from build123d import *

# Parameters (mm, degrees)
SKETCH1_R           = 1.5
SKETCH1_W           = 13
SKETCH1_H           = 19.3
BOSS_EXTRUDE1_DEPTH = 1
FILLET1_R           = 3


with BuildPart() as part:
    # Sketch1 → Boss-Extrude1 (new, symmetric)
    with BuildSketch(Plane(origin=(0, 0, 0), x_dir=(1, 0, 0), z_dir=(0, 1, 0))):
        with BuildLine():
            Line((-105.5, 65), (-105.5, 69))
            ThreePointArc((-105.5, 69), (-109, 72.5), (-112.5, 69))
            Line((-112.5, 69), (-112.5, 65))
            Line((-112.5, 65), (-112.5, -65))
            Line((-112.5, -65), (-112.5, -69))
            ThreePointArc((-112.5, -69), (-109, -72.5), (-105.5, -69))
            Line((-105.5, -69), (-105.5, -65))
            Line((-105.5, -65), (15.5, -65))
            Line((15.5, -65), (15.5, -69))
            ThreePointArc((15.5, -69), (19, -72.5), (22.5, -69))
            Line((22.5, -69), (22.5, -65))
            Line((22.5, -65), (105.5, -65))
            Line((105.5, -65), (105.5, -69))
            ThreePointArc((105.5, -69), (109, -72.5), (112.5, -69))
            Line((112.5, -69), (112.5, -65))
            Line((112.5, -65), (112.5, 65))
            Line((112.5, 65), (112.5, 69))
            ThreePointArc((112.5, 69), (109, 72.5), (105.5, 69))
            Line((105.5, 69), (105.5, 65))
            Line((105.5, 65), (22.5, 65))
            Line((22.5, 65), (22.5, 69))
            ThreePointArc((22.5, 69), (19, 72.5), (15.5, 69))
            Line((15.5, 69), (15.5, 65))
            Line((15.5, 65), (-105.5, 65))
        make_face()
        with Locations(Location((-109, 69, 0), (0, 0, 270))):
            Circle(SKETCH1_R, mode=Mode.SUBTRACT)
        with Locations(Location((109, 69, 0), (0, 0, 90))):
            Circle(SKETCH1_R, mode=Mode.SUBTRACT)
        with Locations(Location((19, 69, 0), (0, 0, 270))):
            Circle(SKETCH1_R, mode=Mode.SUBTRACT)
        with Locations(Location((19, -69, 0), (0, 0, 90))):
            Circle(SKETCH1_R, mode=Mode.SUBTRACT)
        with Locations(Location((109, -69, 0), (0, 0, 270))):
            Circle(SKETCH1_R, mode=Mode.SUBTRACT)
        with Locations(Location((-109, -69, 0), (0, 0, 90))):
            Circle(SKETCH1_R, mode=Mode.SUBTRACT)
        with Locations((-46.5, 0)):
            Rectangle(SKETCH1_W, SKETCH1_H, mode=Mode.SUBTRACT)
    extrude(amount=BOSS_EXTRUDE1_DEPTH, both=True)

    # Fillet1
    fillet1_edges = [part.edges().sort_by_distance(p)[0] for p in [
        (-105.5, 0, -65),
        (15.5, 0, -65),
        (22.5, 0, -65),
        (105.5, 0, -65),
        (105.5, 0, 65),
        (22.5, 0, 65),
        (15.5, 0, 65),
        (-105.5, 0, 65),
    ]]
    fillet(fillet1_edges, radius=FILLET1_R)


solid = part.part
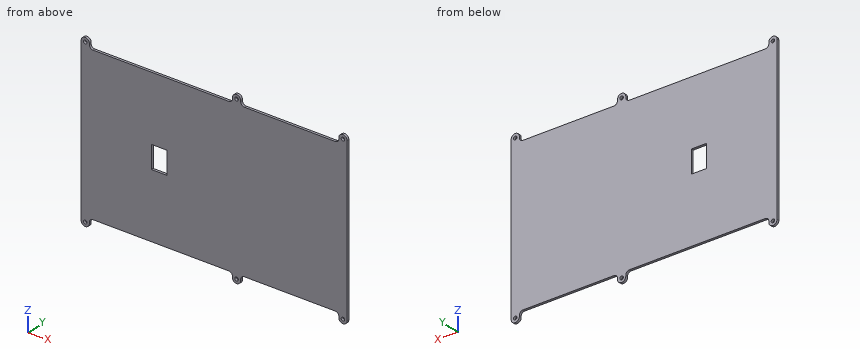
The listing builds one solid part. Answer for the finished solid, in the listing's coordinates (mm). Coordinates: 2 decimals unless noted, no trailing zeros. Loops run counter-clockwise (first coordinate to the right, second up) from the corner with the lowest first, then second, coordinate; pieces in that order, holes last. Notation, with made-up numbers: (2, 74.25) -> (50, 74.25) arc R14 ccw to (50, 95.25) -> close; hole circle Ø2 at (32, 57). An arc over 180 degrees is marked (long way). Answer in a Markdown table with one row per item. Add a question column.
1. Consider line 1 (Z direction, x = -109, y = -0.35); line 2 (X direction, y = 0.1, z = 69); line 3 (X direction, y = -0.5, z = 1.5). Determine where each line is inside the solid, lowest interval first. Write a range as [from, to].
2. The part is cut by section A-A, the plane y = 0.2. Count the separate pieces of the cut face and the enclosed holes in it, then the cut area to 3 significant figures.
3. The part is cut by section B-B, the plane x = 98. Write down the section's boundary in (y, z), then the cut area to 3 significant figures.
4. Flat-ended cylindrical pins translate along their axes: P1, Ø0.6, axis at x = -47.5, y = -0.5, coming from the -Z side; P2, Ø2.5, axis at x = 109, z = -69, coming from the -Y side. Find the tip coordinate at first contact, or state that the pin passes through.
Answer below:
| question | item | result |
|---|---|---|
| 1 | line 1 | [-72.5, -70.5], [-67.5, 67.5], [70.5, 72.5] |
| 1 | line 2 | [-112.5, -110.5], [-107.5, -105.5], [15.5, 17.5], [20.5, 22.5], [105.5, 107.5], [110.5, 112.5] |
| 1 | line 3 | [-112.5, -53], [-40, 112.5] |
| 2 | separate pieces | 1 |
| 2 | enclosed holes | 7 |
| 2 | area | 29,300 mm2 |
| 3 | outline | (-1, -65) -> (1, -65) -> (1, 65) -> (-1, 65) -> close |
| 3 | area | 260 mm2 |
| 4 | P1 | z = -65 |
| 4 | P2 | through |
